Print and shaded views of the part. All mm, measured from the part's lowest x, y and z. A direction names the side the tool comes from. Give positions to 0.01 mm unless a question says otherwise; leave off trailing zeros. Loops run counter-clockwise (first coordinate to the right, second up) from the corner with the lowest first, then second, coordinate; pieces in that order, holes last.
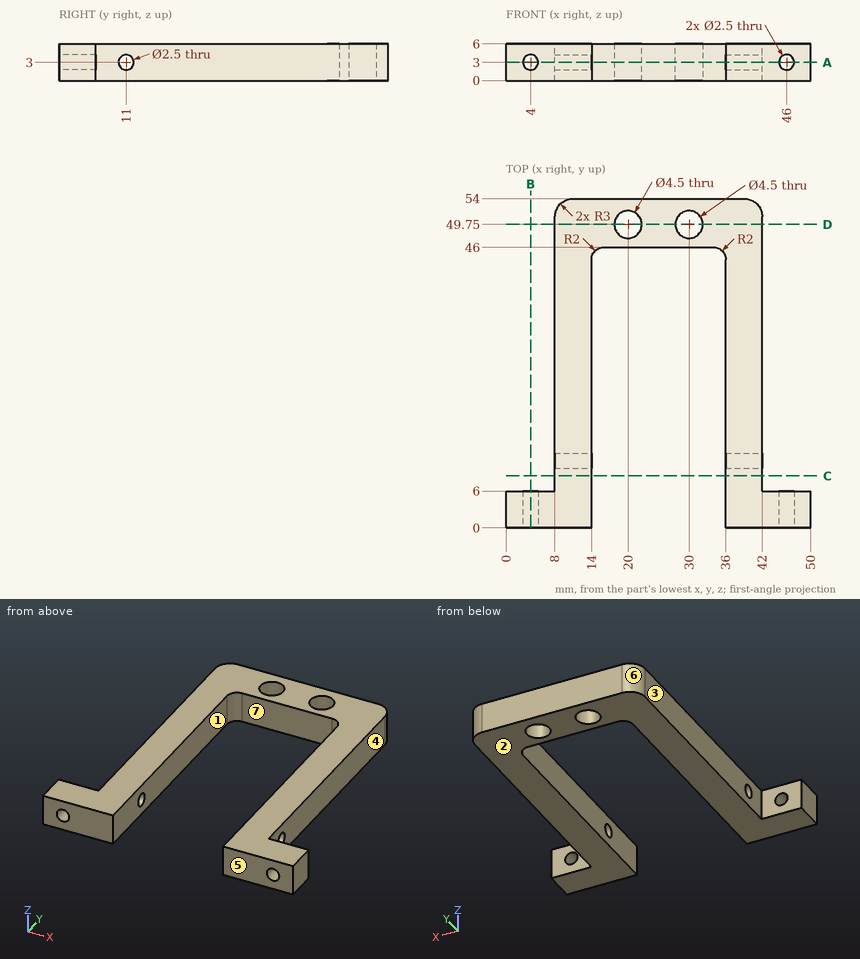
1. Tool access for the marked faces 1, 2, 3 and 4: list every direction of +Z, -Z, +X, -X, +Y, -Y with a clear straight run to the whole face (end or side of a thin tool).
Responses:
face 1: +Z, -Z, -Y
face 2: -Z, +X, -X, +Y, -Y
face 3: +Z, -Z, -X, +Y
face 4: +Z, -Z, +X, +Y
2. Drop flat-ended pins along their axis: pin 1 (5 mm diameter, centred on x = 38, y = 19, fed in from -Z); pin 2 (1.5 mm diameter, centred on y = 27.5, z = 4.5, fed in from -X); pin 3 (5 mm diameter, centred on x = 17.5, y = 35, fed in from +Z); pin 4 (2 mm diameter, centred on y = 48.5, z = 3, fed in from +X). Give the stop position or say it passes through.
Responses:
pin 1: stops at z = 0
pin 2: stops at x = 8
pin 3: passes through
pin 4: stops at x = 42
3. Pull direction X, two halves, no side cores. Call the marked faces 5, 6 and 7: released by +X, released by -X, zero draft, split by the parting line, or undercut.
Responses:
face 5: zero draft
face 6: released by -X
face 7: undercut
4. Saw through at A-A, the plane z = 3. Count the separate pieces of the cut face and the enclosed holes in it, and give its area (3 significant figures).
Responses:
separate pieces: 5
enclosed holes: 2
area: 826 mm2
5. Probe line 1 along X through (y, z) = (18.5, 4.9); line 2 along Z through (x, y) = (46, 1.45); line 3 along Y through (x, z) = (20, 3.1). List the from-to ranges inside material, lowest first.
Responses:
line 1: x = 8 to 14, 36 to 42
line 2: z = 0 to 1.75, 4.25 to 6
line 3: y = 46 to 47.5, 52 to 54
6. Saw through at D-D, the plane y = 49.75. List the corners of the cut face in (x, z), and give its area (3 significant figures).
Responses:
outline: (8, 0) - (17.75, 0) - (17.75, 6) - (8, 6) - close; (22.25, 0) - (27.75, 0) - (27.75, 6) - (22.25, 6) - close; (32.25, 0) - (42, 0) - (42, 6) - (32.25, 6) - close
area: 150 mm2
7. Saw through at B-B, the plane x = 4. List the corners of the cut face in (y, z).
Responses:
outline: (0, 0) - (6, 0) - (6, 1.75) - (0, 1.75) - close; (0, 4.25) - (6, 4.25) - (6, 6) - (0, 6) - close
8. Saw through at C-C, the plane y = 8.5. List the corners of the cut face in (x, z), and give its area (3 significant figures).
Responses:
outline: (8, 0) - (14, 0) - (14, 6) - (8, 6) - close; (36, 0) - (42, 0) - (42, 6) - (36, 6) - close
area: 72.0 mm2
